Job drawing, mm, ordinate dimensions from the low corner. One solid piece. A direction names the side the tool comes from. Coordinates: 2 decimals unless noted, no trailing zeros. Loops run counter-clockwise (first coordinate to the right, second up) from the corner with the lowest first, then second, coordinate; pieces in that order, holes last. Notation, with made-up numbers: (5, 54) -> (41, 54) arc R10 cw to (41, 61) -> close; hole circle Ø7 at (62.25, -21). An arc over 180 degrees is marked (long way). Answer as CSV lines item,"result". Start each with the question number.
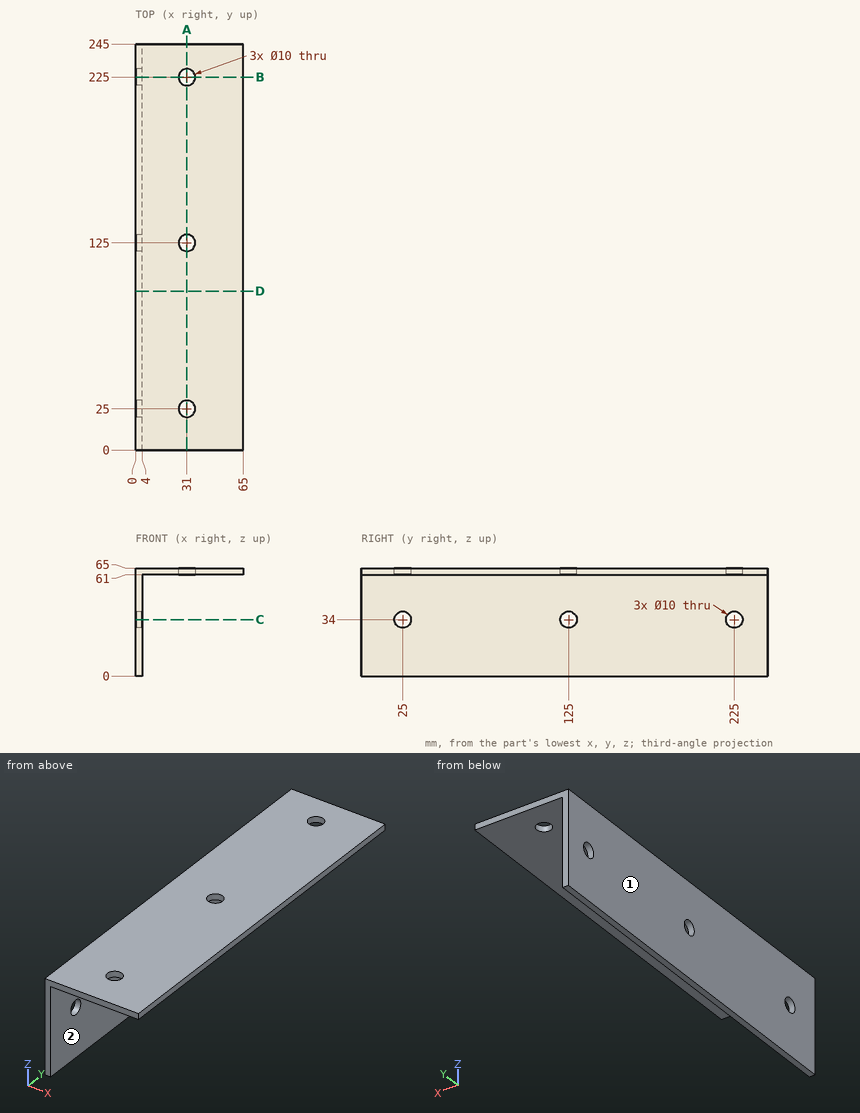
Item 1: Saw through at D-D (y = 96). Write the cut outline in (x, z), plus the area to 3 significant figures.
Item 2: Flat gauge pins, fed straight in: pin 1 Ø4 at (y, z) = (103, 26.5) entering from -X; pin 2 Ø18.5 at (y, z) = (172.5, 17.5) entering from +X; pin 3 Ø1.5 at (x, y) = (30, 174) entering from -Z. Where does each tip first touch, or does it go through?
Item 3: Saw through at B-B (y = 225). Write the cut outline in (x, z), plus the area to 3 significant figures.
Item 4: Saw through at A-A (x = 31). Write the cut outline in (y, z).
Item 5: Saw through at C-C (z = 34). Write the cut outline in (x, y).
Item 6: Wall check: probe 1 along Y at (x, z) = (31, 63); probe 2 along Z at (x, y) = (11, 50); probe 3 along X at (y, z) = (145.5, 56.5). Give the ranges that are in metal, low to high.
Item 7: Which spindle directions (+Z, -Z, +X, -X, +Y, -Y) get a long thin tool onto all of the face, cutting with end or side? Do the marked faces 1 and 2. Say none if no direction does.
Geometry check:
1,outline,"(0, 0) -> (4, 0) -> (4, 61) -> (65, 61) -> (65, 65) -> (0, 65) -> close"
1,area,"504 mm2"
2,pin 1,"x = 0"
2,pin 2,"x = 4"
2,pin 3,"z = 61"
3,outline,"(0, 0) -> (4, 0) -> (4, 29) -> (0, 29) -> close; (0, 39) -> (4, 39) -> (4, 61) -> (26, 61) -> (26, 65) -> (0, 65) -> close; (36, 61) -> (65, 61) -> (65, 65) -> (36, 65) -> close"
3,area,"424 mm2"
4,outline,"(0, 61) -> (20, 61) -> (20, 65) -> (0, 65) -> close; (30, 61) -> (120, 61) -> (120, 65) -> (30, 65) -> close; (130, 61) -> (220, 61) -> (220, 65) -> (130, 65) -> close; (230, 61) -> (245, 61) -> (245, 65) -> (230, 65) -> close"
5,outline,"(0, 0) -> (4, 0) -> (4, 20) -> (0, 20) -> close; (0, 30) -> (4, 30) -> (4, 120) -> (0, 120) -> close; (0, 130) -> (4, 130) -> (4, 220) -> (0, 220) -> close; (0, 230) -> (4, 230) -> (4, 245) -> (0, 245) -> close"
6,probe 1,"0 to 20, 30 to 120, 130 to 220, 230 to 245"
6,probe 2,"61 to 65"
6,probe 3,"0 to 4"
7,face 1,"+Z, -Z, -X, +Y, -Y"
7,face 2,"-Z, +X, +Y, -Y"
